Verification items for this drawing (mm, ordinates from the low corner). A direction names the side the tool comes from. Coordinates: 2 decimals unless noted, no trailing zeros. Write each loop counter-clockwise with the first axis right and the second up, starting at its lowest first coordinate (ties: lowest second). Pieces come first, ordered by that corner, then holes. Notation, with made-up numbers: (43.5, 12.5) -> (75.5, 12.5) arc R13 cw to (75.5, 33.5) -> close; hole circle Ø2 at (-9, 47.25). An arc over 180 degrees is marked (long way). One line per item, written item: value. Start each with the question number.
1) Set-up check for the marked faces 1 and 2: record each of +Z, -Z, +X, -X, +Y, -Y from which the full face is reachable in a straight line by a thin tool's end or side.
2) Sectioned sample at A-A on z = 12.7. Enter the section's corners in (x, y).
3) Sectioned sample at C-C on y = 26. Enter the section's corners in (x, z).
4) Sectioned sample at B-B on x = 10. Enter the section's corners in (y, z).
5) Sectioned sample at D-D on x = 17.25. Enter the section's corners in (y, z), plus the area to 3 significant figures.
6) Gauge pin test, flat ends, axial feed: P1, Ø1.5, axis at x = 10.5, y = 7.5, coming from the -Z side; P2, Ø1.5, axis at x = 4, y = 18.5, coming from the -Z side; P3, Ø10, axis at x = 6, y = 27.5, coming from the -Z side. Record the tip position at first contact, or that the pin passes through.
7) Scan lines: line 1 along Y through (x, z) = (24, 12); line 2 along Z through (x, y) = (12.75, 15). Record each from-to range of solid material in increasing order. Write a range as [from, to].
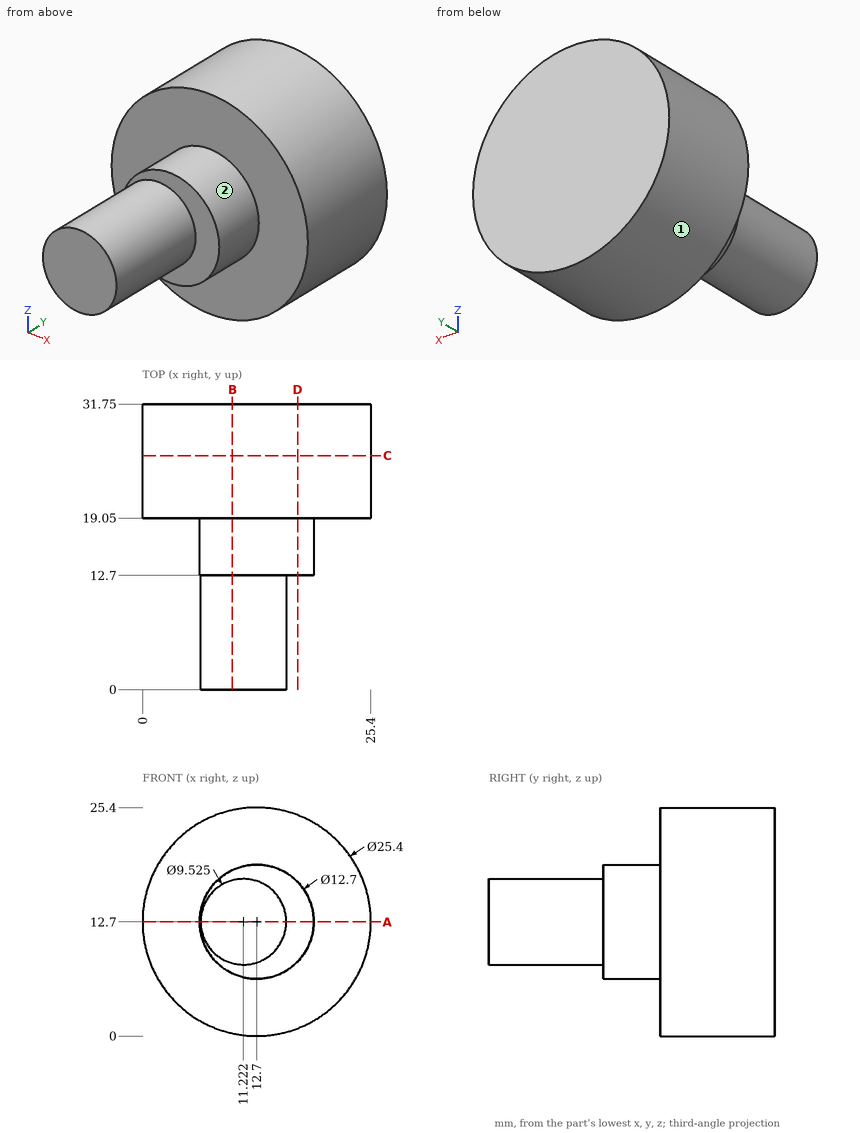
Answers:
1. face 1: +Y, -Y
1. face 2: -Y
2. outline: (0, 19.05) -> (6.35, 19.05) -> (6.35, 12.7) -> (6.46, 12.7) -> (6.46, 0) -> (15.98, 0) -> (15.98, 12.7) -> (19.05, 12.7) -> (19.05, 19.05) -> (25.4, 19.05) -> (25.4, 31.75) -> (0, 31.75) -> close
3. outline: circle Ø25.4 at (12.7, 12.7)
4. outline: (0, 8.1) -> (12.7, 8.1) -> (12.7, 6.95) -> (19.05, 6.95) -> (19.05, 0.29) -> (31.75, 0.29) -> (31.75, 25.11) -> (19.05, 25.11) -> (19.05, 18.45) -> (12.7, 18.45) -> (12.7, 17.3) -> (0, 17.3) -> close
5. outline: (12.7, 8.27) -> (19.05, 8.27) -> (19.05, 0.84) -> (31.75, 0.84) -> (31.75, 24.56) -> (19.05, 24.56) -> (19.05, 17.13) -> (12.7, 17.13) -> close
5. area: 357 mm2
6. P1: stops at z = 7.94
6. P2: stops at z = 2.99
6. P3: stops at z = 0.11
7. line 1: y = [19.05, 31.75]
7. line 2: z = [6.35, 19.05]
